Input: part model. Units: mm. Frame: model coordinates. Round coordinates to 2 decimals unless told otherwise and drop trailing zeros. Loops run counter-clockwise (first coordinate to the right, second up) from the corner with the lowest first, then second, coordinate; pieces in that order, holes last. Notation, with made-up numbers: (73.5, 80.25) -> (117.5, 80.25) arc R12 cw to (117.5, 103.25) -> close; hole circle Ø5 at (4, -14). An arc over 180 degrees is marked (long way). Answer as a JSON object with one key per item and string values. Group by question number.
Item 1: Section query B-B on x = 7.5. Return loops of the section in (y, z).
Item 2: Section query D-D on y = 5. Return loops of the section in (x, z).
Item 3: Section query A-A on z = 0.8. Return loops of the section in (x, y), and give its area (3 significant figures).
Item 4: Material intervals for line 1 (Y direction, x = 8, z = 0.5); line 2 (X direction, y = -5.25, z = 0.55); line 3 (Y direction, x = 11.75, z = 0.1), sorted ascending. Write a range as [from, to].
Item 5: Section query C-C on x = 5.75. Return loops of the section in (y, z).
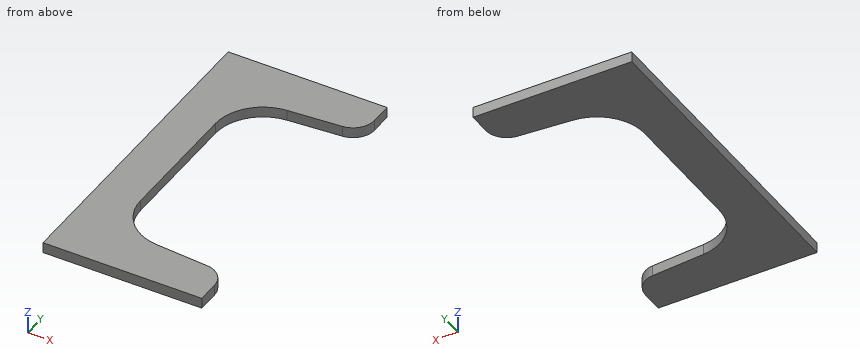
Autodesk Inventor part; units mm, degrees
ref_plane "Начальная плоскость" through (0, 0, 0) normal (0, 0, 1) x (1, 0, 0)
ref_plane "Конечная плоскость" through (0, 0, 1) normal (0, 0, 1) x (1, 0, 0)
ref_plane "YZ Plane" through (0, 0, 0) normal (1, 0, 0) x (0, 1, 0)
ref_plane "Начальная плоскость" through (0, 0, 0) normal (0, 0, 1) x (1, 0, 0)
ref_plane "Конечная плоскость" through (0, 0, 1) normal (0, 0, 1) x (1, 0, 0)
sketch "Эскиз" plane through (0, 0, 0) normal (0, 0, 1) x (1, 0, 0)
  line L0 (0, -15) -> (0, 15)
  line L1 (0, 15) -> (15, 15)
  line L2 (15, 15) -> (15, 12.9464)
  line L3 (13.1595, 10.9528) -> (8.1411, 10.5513)
  line L4 (4, 6.0656) -> (4, -6.0656)
  line L5 (7.5, 15) -> (7.5, 10.5) construction
  line L6 (15, 11.1) -> (15, 10.5) construction
  line L7 (15, 10.5) -> (7.5, 10.5) construction
  line L8 (0, -15) -> (15, -15)
  line L9 (15, -15) -> (15, -12.9464)
  line L10 (13.1595, -10.9528) -> (8.1411, -10.5513)
  arc A0 (8.1411, 10.5513) -> (4, 6.0656) centre (8.5, 6.0656) ccw
  arc A1 (4, -6.0656) -> (8.1411, -10.5513) centre (8.5, -6.0656) ccw
  arc A2 (13.1595, 10.9528) -> (15, 12.9464) centre (13, 12.9464) ccw
  arc A3 (15, -12.9464) -> (13.1595, -10.9528) centre (13, -12.9464) ccw
  line L11 (0, 0) -> (4, 0) construction
  line L12 (0, 0) -> (15, 0) construction
  point P0 (7.5, -10.5)
  dimension "d5" = 0.6
  dimension "d23" = 4.5
  dimension "d24" = 2
  dimension "d31" = 15
  dimension "d32" = 7.5
  dimension "d33" = 4.5
  dimension "d34" = 30
  dimension "d35" = 4
  dimension "d36" = 7.5
  dimension "d37" = 4.5
  dimension "d38" = 90
extrude "Базовый элемент" add sketch "Эскиз" along normal up to surface (1 mm away) from surface at 0
sketch "Sketch3" plane through (0, 0, 0) normal (0, 0, 1) x (1, 0, 0)
  line L0 (0, 0) -> (10, 0)
ref_plane "Work Plane3" through (0, 0, 0) normal (0, -1, 0) x (1, 0, 0)
sketch "Sketch4" plane through (0, 0, 0) normal (0, -1, 0) x (1, 0, 0)
  line L0 (-2, 0) -> (12, 0)
  line L1 (-2, 1) -> (12, 1)
  dimension "d29" = 1
equation "\"d23\" = G_IR"
equation "\"d24\" = G_ER"
equation "\"d31\" = G_W"
equation "\"d32\" = G_C"
equation "\"d33\" = G_T1"
equation "\"d34\" = G_H"
equation "\"d35\" = G_T"
equation "\"d6\" = G_L"
equation "\"G_W\" = 15"
equation "\"G_H\" = 30"
equation "\"G_T\" = 4"
equation "\"G_T1\" = 4.5"
equation "\"G_NG\" = 0.08"
equation "\"G_ER\" = 2"
equation "\"G_IR\" = 4.5"
equation "\"G_C\" = 7.5"
equation "\"G_L\" = d29"
equation "\"ex\" = 0"
equation "\"G_OFFSET_START\" = 0"
equation "\"G_OFFSET_END\" = 0"
equation "\"d27\" = G_OFFSET_END + B_L"
equation "\"B_L\" = 1"
properties part number "DIN 1026-1" material "S235JR ДСТУ EN 10025-1"
Solved:
{
 "1": {"outline": "(-15, 0) -> (-10.45, 0) -> (-10.45, 1) -> (-15, 1) -> close; (10.45, 0) -> (15, 0) -> (15, 1) -> (10.45, 1) -> close"},
 "2": {"outline": "(0, 0) -> (4, 0) -> (4, 1) -> (0, 1) -> close"},
 "3": {"outline": "(0, -15) -> (15, -15) -> (15, -12.95) arc R2 ccw to (13.16, -10.95) -> (8.14, -10.55) arc R4.5 cw to (4, -6.07) -> (4, 6.07) arc R4.5 cw to (8.14, 10.55) -> (13.16, 10.95) arc R2 ccw to (15, 12.95) -> (15, 15) -> (0, 15) -> close", "area": "221 mm²"},
 "4": {"line 1": "[-15, -10.54], [10.54, 15]", "line 2": "[0, 4]", "line 3": "[-15, -10.84], [10.84, 15]"},
 "5": {"outline": "(-15, 0) -> (-9.63, 0) -> (-9.63, 1) -> (-15, 1) -> close; (9.63, 0) -> (15, 0) -> (15, 1) -> (9.63, 1) -> close"}
}
